from build123d import *

# Parameters (mm, degrees)
SKETCH1_W           = 129.794
SKETCH1_H           = 24.384
BOSS_EXTRUDE1_DEPTH = 5.334
SKETCH3_W           = 58.42
SKETCH3_H           = 18.034
CUT_EXTRUDE1_DEPTH  = 104.917980915
SKETCH6_W           = 38.1
SKETCH6_H           = 5.334
BOSS_EXTRUDE2_DEPTH = 8.89
SKETCH7_W           = 5.08
SKETCH7_H           = 5.08
CUT_EXTRUDE4_DEPTH  = 104.917980915
SKETCH8_W           = 8.89
SKETCH8_H           = 5.334
CUT_EXTRUDE5_DEPTH  = 104.917980915
SKETCH4_R           = 0.889
CUT_EXTRUDE6_DEPTH  = 104.917980915
SKETCH9_W           = 129.794
SKETCH9_H           = 5.334
BOSS_EXTRUDE3_DEPTH = 2.54


with BuildPart() as part:
    # Sketch1 → Boss-Extrude1 (new body)
    with BuildSketch(Plane.XY):
        with Locations((-20.165445418, -47.262819662)):
            Rectangle(SKETCH1_W, SKETCH1_H)
    extrude(amount=BOSS_EXTRUDE1_DEPTH)

    # Sketch3 → Cut-Extrude1 (cut, through all)
    with BuildSketch(Plane.XY.offset(5.334)):
        with Locations((-22.578445418, -44.087819662)):
            Rectangle(SKETCH3_W, SKETCH3_H)
    extrude(amount=-CUT_EXTRUDE1_DEPTH, mode=Mode.SUBTRACT)

    # Sketch6 → Boss-Extrude2 (add)
    with BuildSketch(Plane(origin=(0, -35.070819662, 0), x_dir=(1, 0, 0), z_dir=(0, 1, 0))):
        with Locations((25.681554582, -2.667)):
            Rectangle(SKETCH6_W, SKETCH6_H)
    extrude(amount=BOSS_EXTRUDE2_DEPTH)

    # Sketch7 → Cut-Extrude4 (cut, through all)
    with BuildSketch(Plane.XY.offset(5.334)):
        with Locations((42.191554582, -28.720819662)):
            Rectangle(SKETCH7_W, SKETCH7_H)
    extrude(amount=-CUT_EXTRUDE4_DEPTH, mode=Mode.SUBTRACT)

    # Sketch8 → Cut-Extrude5 (cut, through all)
    with BuildSketch(Plane.XY.offset(5.334)):
        with Locations((25.681554582, -41.547819662)):
            Rectangle(SKETCH8_W, SKETCH8_H)
    extrude(amount=-CUT_EXTRUDE5_DEPTH, mode=Mode.SUBTRACT)

    # Sketch4 → Cut-Extrude6 (cut, through all)
    with BuildSketch(Plane.XY.offset(5.334)):
        with Locations((-56.995445418, -43.325819662)):
            Circle(SKETCH4_R)
    extrude(amount=-CUT_EXTRUDE6_DEPTH, mode=Mode.SUBTRACT)

    # Sketch9 → Boss-Extrude3 (add)
    with BuildSketch(Plane(origin=(0, -59.454819662, 0), x_dir=(-1, 0, 0), z_dir=(0, -1, 0))):
        with Locations((20.165445418, -2.667)):
            Rectangle(SKETCH9_W, SKETCH9_H)
    extrude(amount=BOSS_EXTRUDE3_DEPTH)


solid = part.part
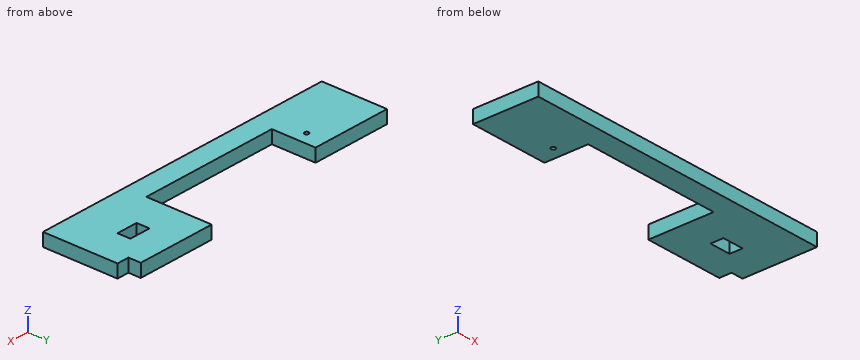
Check sheet for the modelled part. Datum: model origin and axes. Units: mm. Round coordinates to 2 decimals unless told otherwise and drop trailing zeros. Order: outer loops, then holes, each group sorted by start corner. A loop starts at its lowest first (then second) coordinate and runs counter-clockwise, first axis right, second up.
Q1. Cross-section at A-A, the plane x = 25.5. Enter the section's corners in (y, z), plus the area to 3 significant figures.
Filled sheet:
outline: (-61.99, 0) - (-44.21, 0) - (-44.21, 5.33) - (-61.99, 5.33) - close; (-38.88, 0) - (-26.18, 0) - (-26.18, 5.33) - (-38.88, 5.33) - close
area: 163 mm2
Q2. Scan lines: L1, parallel to X at y = -48, z = 0.95; L2, parallel to X at y = -28.5, z = 2.4; L3, parallel to Y at x = 6, z = 1.3. Record each from-to range of solid material in increasing order.
Filled sheet:
L1: x = -85.06 to -51.79, 6.63 to 44.73
L2: x = 6.63 to 39.65
L3: y = -61.99 to -53.1
Q3. Cross-section at B-B, the plane y = -36.5. Enter the section's corners in (x, z).
Filled sheet:
outline: (-85.06, 0) - (-51.79, 0) - (-51.79, 5.33) - (-85.06, 5.33) - close; (6.63, 0) - (44.73, 0) - (44.73, 5.33) - (6.63, 5.33) - close
Q4. Cross-section at D-D, the plane x = -75.5. Enter the section's corners in (y, z).
Filled sheet:
outline: (-61.99, 0) - (-35.07, 0) - (-35.07, 5.33) - (-61.99, 5.33) - close
Q5. Cross-section at C-C, the plane z = 0.95. Enter the section's corners in (x, y), plus the area to 3 significant figures.
Filled sheet:
outline: (-85.06, -61.99) - (44.73, -61.99) - (44.73, -31.26) - (39.65, -31.26) - (39.65, -26.18) - (6.63, -26.18) - (6.63, -53.1) - (-51.79, -53.1) - (-51.79, -35.07) - (-85.06, -35.07) - close; hole circle Ø1.78 at (-57, -43.33); hole (21.24, -44.21) - (30.13, -44.21) - (30.13, -38.88) - (21.24, -38.88) - close
area: 2,700 mm2
